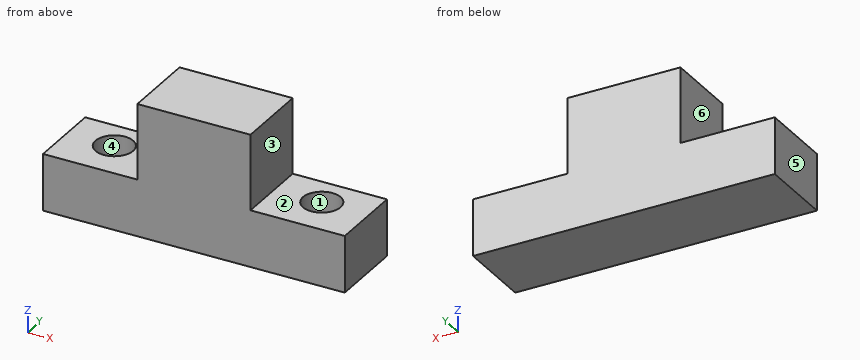
from build123d import *

# Parameters (mm, degrees)
F1_DEPTH = 25.4
F2_R     = 6.35
F3_DEPTH = 12.7


with BuildPart() as f1:
    # F0 (on Front) → F1 (new body)
    with BuildSketch(Plane.XZ):
        Polygon((0, 0), (-19.05, 0), (-19.05, -25.4), (-50.8, -25.4), (-50.8, -44.45), (0, -44.45), align=None)
    extrude(amount=F1_DEPTH)

    # F2 (on face) → F3 (cut)
    with BuildSketch(Plane.XY.offset(-25.4)):
        with Locations((-34.925, -10.856094)):
            Circle(F2_R)
    extrude(amount=-F3_DEPTH, mode=Mode.SUBTRACT)

    # F4: F1 across plane


with BuildPart() as f1_1:
    add(f1.part)
    add(f1.part.mirror(Plane.YZ))


solid = f1_1.part
The listing builds one solid part. Answer for the finished solid, in the listing's coordinates (mm). Face numbers are marked on the shaded views. A direction names the side the tool comes from. Give positions to 0.01 mm unless a question says otherwise; leave off trailing zeros. Write each loop counter-clockwise with the first axis right and the second up, starting at its lowest first coordinate (ties: lowest second). Pieces come first, ordered by that corner, then holes. Notation, with made-up numbers: (60.25, -23.75) - (84.25, -23.75) arc R24 cw to (84.25, 9.25) - close; hole circle Ø10 at (48.25, 75.5). An arc over 180 degrees is marked (long way). One line per question, with ' | ' between items. Start each with the question number.
1. Determine the mould class of the marked faces 1, 2, 3 and 4 for opening direction X: +X half, -X half, draft (parallel to the pull), parting line (faces both ways), or undercut.
2. Section B-B, the plane z = -8 is taken. Determine the outline of the cut face in (x, y), then the cut area to 3 significant figures.
3. Section A-A, the plane y = -20.5 is taken. Determine the outline of the cut face in (x, z), then the cut area to 3 significant figures.
4. Section C-C, the plane x = -35 is taken. Determine the outline of the cut face in (y, z).
5. Given P1, Ø10, axis at x = -34.92, y = -10.86, coming from the +Z side; P2, Ø8, axis at y = -13, z = -18, coming from the +X side; P3, Ø6, axis at x = 3.5, z = -25.5, coming from the +Y side; P4, Ø14, axis at x = 38, y = -10.5, coming from the +Z side, each flat-ended and moving along its own axis, determine where each tip first touches the part or whether it passes through.
6. Section D-D, the plane z = -34.5 is taken. Determine the outline of the cut face in (x, y) (3 decimals).
7. Straight lines are drawn through the part: line 1 (X direction, y = -5.25, z = -27); line 2 (X direction, y = -6.5, z = -25); line 3 (Z direction, x = -29, y = -21.75). For each, find the intervals that lie inside material, in ascending order.
8. For the marked faces 5 and 6, determine the directions among +Z, -Z, +X, -X, +Y, -Y from which every point of the face is accessible in a straight line to the end or side of a thin tool.
Result:
1) face 1: undercut | face 2: draft | face 3: +X half | face 4: undercut
2) outline: (-19.05, -25.4) - (19.05, -25.4) - (19.05, 0) - (-19.05, 0) - close | area: 968 mm2
3) outline: (-50.8, -44.45) - (50.8, -44.45) - (50.8, -25.4) - (19.05, -25.4) - (19.05, 0) - (-19.05, 0) - (-19.05, -25.4) - (-50.8, -25.4) - close | area: 2,900 mm2
4) outline: (-25.4, -44.45) - (0, -44.45) - (0, -25.4) - (-4.51, -25.4) - (-4.51, -38.1) - (-17.21, -38.1) - (-17.21, -25.4) - (-25.4, -25.4) - close
5) P1: stops at z = -38.1 | P2: stops at x = 19.05 | P3: stops at y = 0 | P4: stops at z = -25.4
6) outline: (-50.8, -25.4) - (50.8, -25.4) - (50.8, 0) - (-50.8, 0) - close; hole circle Ø12.7 at (-34.925, -10.856); hole circle Ø12.7 at (34.925, -10.856)
7) line 1: x = -50.8 to -37.91, -31.94 to 31.94, 37.91 to 50.8 | line 2: x = -19.05 to 19.05 | line 3: z = -44.45 to -25.4
8) face 5: +Z, -Z, -X, +Y, -Y | face 6: +Z, -X, +Y, -Y
